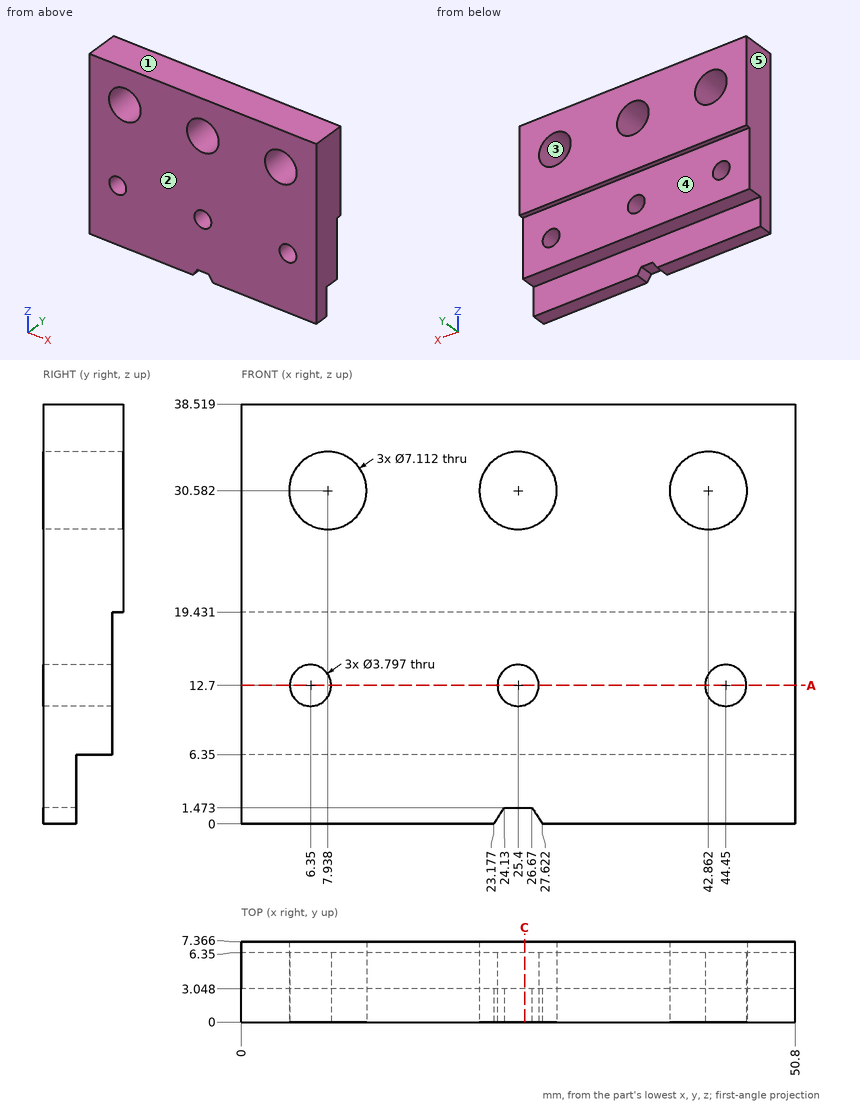
Study the drawing (mm; zero at the part's minimum x, y, z) and answer. A direction names the side the tool comes from. Round coordinates to 2 decimals unless told otherwise and drop trailing zeros. Write each loop counter-clockwise with the first axis right and the second up, starting at its lowest first coordinate (ties: lowest second). Pieces come first, ordered by that corner, then holes. Notation, with made-up numbers: (77, 63.25) -> (96, 63.25) arc R10 ccw to (96, 70.25) -> close; hole circle Ø6 at (85.25, 44.5). An arc over 180 degrees is marked (long way). Use CSV: the item, a comma, the result in double quotes. Start each with the question number.
(1) Section A-A on z = 12.7 is taken. Give the vertices of the cut face in (x, y), then the cut area to 3 significant figures.
(2) Section C-C on x = 26 is taken. Count the separate pieces of the cut face and the enclosed holes in it, then the cut area to 3 significant figures.
(3) Which of the six approach directions +Z, -Z, +X, -X, +Y, -Y give full straight-line access (tool end or side, diameter ignored) to the marked faces 4 and 5?
(4) Consider L1, parallel to X at y = 2.25, z = 33.5 (1 decimal); L2, parallel to Z at x = 25.4, y = 2.25 (1 decimal); L3, parallel to X at y = 3.5, z = 14 (1 decimal). Determine where each line is inside the solid, lowest interval first. Write a range as from..to.
(5) Each of these flat-tipped pins is pushed along its axis until it touches: pin 1 (5.5 mm diameter, centred on x = 42.86, z = 30.58, fed in from +Y); pin 2 (14.5 mm diameter, centred on x = 35, z = 11.5, fed in from +Y); pin 3 (1.1 mm diameter, centred on x = 27.5, y = 7, fed in from -Z); pin 4 (1.9 mm diameter, centred on x = 20.5, z = 4, fed in from +Y). Where does it stop, or does it pass through?
(6) The mould has two halves that part along Z. Classify the marked faces 1, 2 and 3: released by +Z, released by -Z, zero draft, split by the parting line, or undercut.
A:
1,outline,"(0, 0) -> (4.45, 0) -> (4.45, 6.35) -> (0, 6.35) -> close; (8.25, 0) -> (23.5, 0) -> (23.5, 6.35) -> (8.25, 6.35) -> close; (27.3, 0) -> (42.55, 0) -> (42.55, 6.35) -> (27.3, 6.35) -> close; (46.35, 0) -> (50.8, 0) -> (50.8, 6.35) -> (46.35, 6.35) -> close"
1,area,"250 mm²"
2,separate pieces,"3"
2,enclosed holes,"0"
2,area,"164 mm²"
3,face 4,"-Z, +X, -X, +Y"
3,face 5,"+Z, -Z, -X, +Y, -Y"
4,L1,"x = 0..5.9, 10..23.4, 27.4..40.8, 44.9..50.8"
4,L2,"z = 1.5..10.8, 14.6..27, 34.1..38.5"
4,L3,"x = 0..5, 7.7..24, 26.8..43.1, 45.8..50.8"
5,pin 1,"passes through"
5,pin 2,"stops at y = 6.35"
5,pin 3,"stops at z = 19.43"
5,pin 4,"stops at y = 3.05"
6,face 1,"released by +Z"
6,face 2,"zero draft"
6,face 3,"undercut"
